Check sheet for the modelled part. Datum: model origin and axes. Units: mm. A direction names the side the tool comes from. Coordinates: 2 decimals unless noted, no trailing zeros. Loops run counter-clockwise (first coordinate to the right, second up) from the corner with the lowest first, then second, coordinate; pieces in that order, holes last. Notation, with made-up numbers: (7.25, -20) -> (49.25, -20) arc R18 cw to (49.25, 0) -> close; hole circle Ø9 at (87, 59). An arc over 180 degrees is marked (long way). Use CSV: the item, a comma, the result in double quotes.
```python
from build123d import *

# Parameters (mm, degrees)
SKETCH2_W           = 30
SKETCH2_H           = 30
SKETCH2_R           = 1.6
BOSS_EXTRUDE1_DEPTH = 9.25
SKETCH3_W           = 3.25
SKETCH3_H           = 25
CUT_EXTRUDE1_DEPTH  = 44.423064148
SKETCH5_W           = 30
SKETCH5_H           = 3
BOSS_EXTRUDE2_DEPTH = 11


with BuildPart() as part:
    # Sketch2 → Boss-Extrude1 (new body)
    with BuildSketch(Plane(origin=(0, 0, 0), x_dir=(0, 0, -1), z_dir=(1, 0, 0))):
        with Locations((15, 15)):
            Rectangle(SKETCH2_W, SKETCH2_H)
        with Locations((5, 10)):
            Circle(SKETCH2_R, mode=Mode.SUBTRACT)
        with Locations((25, 10)):
            Circle(SKETCH2_R, mode=Mode.SUBTRACT)
    extrude(amount=-BOSS_EXTRUDE1_DEPTH)

    # Sketch3 → Cut-Extrude1 (cut, through all)
    with BuildSketch(Plane.XY):
        with Locations((-4.625, 12.5)):
            Rectangle(SKETCH3_W, SKETCH3_H)
    extrude(amount=-CUT_EXTRUDE1_DEPTH, mode=Mode.SUBTRACT)

    # Sketch5 → Boss-Extrude2 (add)
    with BuildSketch(Plane.ZY.offset(9.25)):
        with Locations((-15, 28.5)):
            Rectangle(SKETCH5_W, SKETCH5_H)
    extrude(amount=BOSS_EXTRUDE2_DEPTH)


solid = part.part
```
1) Cross-section at D-D on z = -8.5. Record the boundary of the cut face in (x, y), and give its area (3 significant figures).
Answer below:
outline,"(-20.25, 27) -> (-9.25, 27) -> (-9.25, 0) -> (-6.25, 0) -> (-6.25, 25) -> (-3, 25) -> (-3, 0) -> (0, 0) -> (0, 30) -> (-20.25, 30) -> close"
area,"229 mm²"
2) Draft check along Z on faces 4 (the cylindrical face through (-7.73, 8.44, -4.65)), 5 (the cylindrical face through (-1.48, 8.44, -24.65)), 6 (the flat face through (-7, 18, 0)), 7 (the flat face through (-8, 0, -15)). Enter one of: released by +Z, released by -Z, zero draft, split by the parting line, or undercut.
Answer below:
face 4,"undercut"
face 5,"undercut"
face 6,"released by +Z"
face 7,"zero draft"
3) Go/stop test with flat-tipped pins: pin 1 Ø10 at (x, z) = (-15, -9) entering from -Y; pin 2 Ø13.5 at (y, z) = (7, -21.5) entering from -X; pin 3 Ø1.6 at (x, z) = (-4.5, -10) entering from -Y. Record where each tip stops, or that it passes through.
Answer below:
pin 1,"stops at y = 27"
pin 2,"stops at x = -9.25"
pin 3,"stops at y = 25"
4) Thickness scan on line 1 along X through (y, z) = (16.5, -2.75); line 2 along Y through (x, z) = (-8.1, -25); line 3 along Y through (x, z) = (-11, -19). Record the ranges inside material, lowest first. Write a range as from..to.
Answer below:
line 1,"x = -9.25..-6.25, -3..0"
line 2,"y = 0..8.4, 11.6..30"
line 3,"y = 27..30"
5) Cross-section at C-C on z = -25. Record the boundary of the cut face in (x, y).
Answer below:
outline,"(-20.25, 27) -> (-9.25, 27) -> (-9.25, 11.6) -> (-6.25, 11.6) -> (-6.25, 25) -> (-3, 25) -> (-3, 11.6) -> (0, 11.6) -> (0, 30) -> (-20.25, 30) -> close; (-9.25, 0) -> (-6.25, 0) -> (-6.25, 8.4) -> (-9.25, 8.4) -> close; (-3, 0) -> (0, 0) -> (0, 8.4) -> (-3, 8.4) -> close"
6) Access from +Z, -Z, +X, -X, +Y, -Y to the whole of each face (thin tool, end or side, straight path). Record for faces 1 (the flat face through (-7, 18, -30)), 2 (the flat face through (-5, 25, -15)), 3 (the flat face through (-9.25, 14, -15)).
Answer below:
face 1,"-Z, +X, -X, +Y, -Y"
face 2,"+Z, -Z, -Y"
face 3,"+Z, -Z, -X, -Y"
7) Cross-section at B-B on y = 3.75. Record the boundary of the cut face in (x, z).
Answer below:
outline,"(-9.25, -30) -> (-6.25, -30) -> (-6.25, 0) -> (-9.25, 0) -> close; (-3, -30) -> (0, -30) -> (0, 0) -> (-3, 0) -> close"
8) Cross-section at A-A on y = 10. Record the boundary of the cut face in (x, z), and give its area (3 significant figures).
Answer below:
outline,"(-9.25, -30) -> (-6.25, -30) -> (-6.25, -26.6) -> (-9.25, -26.6) -> close; (-9.25, -23.4) -> (-6.25, -23.4) -> (-6.25, -6.6) -> (-9.25, -6.6) -> close; (-9.25, -3.4) -> (-6.25, -3.4) -> (-6.25, 0) -> (-9.25, 0) -> close; (-3, -30) -> (0, -30) -> (0, -26.6) -> (-3, -26.6) -> close; (-3, -23.4) -> (0, -23.4) -> (0, -6.6) -> (-3, -6.6) -> close; (-3, -3.4) -> (0, -3.4) -> (0, 0) -> (-3, 0) -> close"
area,"142 mm²"
